Source: CAD feature listing. Evaluate the final solid. Frame: model axes, mm. A direction names the side the tool comes from. Give positions to 0.01 mm unless a question says otherwise; leave off trailing zeros. Write each loop counter-clockwise with the first axis right and the second up, starting at its lowest first coordinate (ties: lowest second). Pieces come first, ordered by that corner, then holes. Notation, with made-up numbers: (29, 74) - (78, 74) arc R14 cw to (78, 86) - close; hole circle Ø11 at (3.5, 39.5). An arc over 180 degrees is marked (long way). One line per question, with ' | ' between items. Start each with the question number.
(1) Draft query along Y for faces 1 (the flat face through (57, 0, 0)), 2 (the flat face through (155.1, -24.42, 9.86)), 3 (the flat face through (165.99, 18.75, 4.93)). Return one class per face: +Y half, -Y half, draft (parallel to the pull), parting line (faces both ways), or undercut.
(2) Section B-B, the plane y = 0. Return loops of the section in (x, z).
(3) Section D-D, the plane z = 6. Return loops of the section in (x, y), plus the area to 3 significant figures.
(4) Ray query, line 1 (Z direction, x = 47, y = 25); line 2 (Z direction, x = 128.5, y = 8); line 3 (Y direction, x = 100, z = 6). Return the intervals inside material, ascending. Write a range as [from, to].
(5) Section C-C, the plane x = 112. Return loops of the section in (y, z).
(6) Pin query (flat end, axial travel): pin 1 (1.5 mm diameter, centred on x = -8, z = -64, fed in from -Y); pin 2 (8 mm diameter, centred on x = 169, y = 23, fed in from -Z); pin 3 (6 mm diameter, centred on y = 45, z = -23.5, fed in from +X); pin 4 (5 mm diameter, centred on x = 44.5, y = 23.5, fed in from -Z). Return the tip coordinate at first contact, or that it passes through.
(7) Access query for faces 4 (the cylindrical face through (-64.964, 2.173, 9.86)), 5 (the flat face through (-19.72, -34.803, -43.025)). Directions: +Z, -Z, +X, -X, +Y, -Y. A direction counts if a zero-diameter tool reaches every point of the face in a straight line with its end or side. Return the directions, or none.
(8) Section A-A, the plane z = -43.5. Return loops of the section in (x, y), plus the area to 3 significant figures.
```python
from build123d import *

# Parameters (mm, degrees)
BOSS_EXTRUDE1_DEPTH = 20
CUT_EXTRUDE1_DEPTH  = 10
SKETCH9_R           = 50
BOSS_EXTRUDE4_DEPTH = 80
CUT_EXTRUDE4_DEPTH  = 75


with BuildPart() as part:
    # Sketch3 → Boss-Extrude1 (new body)
    with BuildSketch(Plane.XY):
        with BuildLine():
            Line((231.34250824, 19.965947877), (80.967339763, 28.752193652))
            ThreePointArc((80.967339763, 28.752193652), (62.680914893, 33.385308199), (47.412586794, 44.463992326))
            ThreePointArc((47.412586794, 44.463992326), (-65, 0), (47.412586794, -44.463992326))
            ThreePointArc((47.412586794, -44.463992326), (62.680914893, -33.385308199), (80.967339763, -28.752193652))
            Line((80.967339763, -28.752193652), (231.34250824, -19.965947877))
            ThreePointArc((231.34250824, -19.965947877), (250.175921184, 0), (231.34250824, 19.965947877))
        make_face()
    extrude(amount=BOSS_EXTRUDE1_DEPTH)

    # Sketch4 → Cut-Extrude1 (cut)
    with BuildSketch(Plane(origin=(0, 0, 0), x_dir=(-1, 0, 0), z_dir=(0, 0, -1))):
        with BuildLine():
            Line((-231.376219968, -12.442237854), (-102.400597569, -24.884475709))
            ThreePointArc((-102.400597569, -24.884475709), (-75, 0), (-102.400597569, 24.884475709))
            Line((-102.400597569, 24.884475709), (-231.376219968, 12.442237854))
            ThreePointArc((-231.376219968, 12.442237854), (-242.675921184, 0), (-231.376219968, -12.442237854))
        make_face()
    extrude(amount=-CUT_EXTRUDE1_DEPTH, mode=Mode.SUBTRACT)

    # Sketch9 → Boss-Extrude4 (add)
    with BuildSketch(Plane(origin=(0, 0, 0), x_dir=(-1, 0, 0), z_dir=(0, 0, -1))):
        with Locations(Location((0, 0, 0), (0, 0, 180))):
            Circle(SKETCH9_R)
    extrude(amount=BOSS_EXTRUDE4_DEPTH)

    # Sketch10 → Cut-Extrude4 (cut)
    with BuildSketch(Plane(origin=(0, 0, -80), x_dir=(-1, 0, 0), z_dir=(0, 0, -1))):
        Polygon((0, 46.188021535), (-40, 23.094010768), (-40, -23.094010768), (0, -46.188021535), (40, -23.094010768), (40, 23.094010768), align=None)
    extrude(amount=-CUT_EXTRUDE4_DEPTH, mode=Mode.SUBTRACT)


solid = part.part
```
Check sheet entries:
1) face 1: draft | face 2: -Y half | face 3: undercut
2) outline: (-65, 0) - (-50, 0) - (-50, -80) - (-40, -80) - (-40, -5) - (40, -5) - (40, -80) - (50, -80) - (50, 0) - (75, 0) - (75, 10) - (242.68, 10) - (242.68, 0) - (250.18, 0) - (250.18, 20) - (-65, 20) - close
3) outline: (47.41, -44.46) arc R50 cw to (80.97, -28.75) - (231.34, -19.97) arc R20 ccw to (231.34, 19.97) - (80.97, 28.75) arc R50 cw to (47.41, 44.46) arc R65 ccw (long way) to start; hole (102.4, -24.88) - (231.38, -12.44) arc R12.5 ccw to (231.38, 12.44) - (102.4, 24.88) arc R25 ccw (long way) to start | area: 16,300 mm²
4) line 1: [0, 20] | line 2: [10, 20] | line 3: [-27.64, -25], [25, 27.64]
5) outline: (-26.94, 0) - (-23.96, 0) - (-23.96, 10) - (23.96, 10) - (23.96, 0) - (26.94, 0) - (26.94, 20) - (-26.94, 20) - close
6) pin 1: y = -49.47 | pin 2: z = 0 | pin 3: x = 27.13 | pin 4: z = -80
7) face 4: +Z, -Z | face 5: -Z
8) outline: circle Ø100 at (0, 0); hole (-40, -23.09) - (0, -46.19) - (40, -23.09) - (40, 23.09) - (0, 46.19) - (-40, 23.09) - close | area: 2,310 mm²
